```python
from build123d import *

# Parameters (mm, degrees)
SKETCH1_R                = 1.524
SKETCH1_R_2              = 1.27
SKETCH1_R_3              = 0.762
BOSS_EXTRUDE1_DEPTH      = 2.032
SKETCH1_3_R              = 1.27
SKETCH1_3_R_2            = 0.762
CUT_EXTRUDE1_DEPTH       = 1.524
SKETCH3_R                = 1.651
CUT_EXTRUDE2_DEPTH       = 0.254
SKETCH3_3_R              = 1.651
CUT_EXTRUDE3_DEPTH       = 2.032
SKETCH4_R                = 1.9685
BOSS_EXTRUDE2_DEPTH      = 0.254
BOSS_EXTRUDE3_DEPTH      = 2.54
BOSS_EXTRUDE3_DEPTH_BACK = 0.762
SKETCH4_3_R              = 1.9685
SKETCH4_3_R_2            = 1.651
SKETCH4_3_R_3            = 0.762
CUT_EXTRUDE4_DEPTH       = 2.032
SKETCH10_R               = 0.762
BOSS_EXTRUDE4_DEPTH      = 0.2286


with BuildPart() as part:
    # Sketch1 → Boss-Extrude1 (new body)
    # profile 1 of 7: a face of its own
    with BuildSketch(Plane(origin=(0, 0, 0), x_dir=(1, 0, 0), z_dir=(0, 1, 0))):
        with BuildLine():
            Line((2.032, -6.212875778), (2.032, -1.24150214))
            ThreePointArc((2.032, -1.24150214), (0, -2.38125), (-2.032, -1.24150214))
            Line((-2.032, -1.24150214), (-2.032, -6.206396707))
            ThreePointArc((-2.032, -6.206396707), (-0.877113637, -6.887720967), (0.461163405, -6.804175651))
            Line((0.461163405, -6.804175651), (2.032, -6.212875778))
        make_face()
        with Locations((0, -4.318)):
            Circle(SKETCH1_R, mode=Mode.SUBTRACT)
    # profile 2 of 7: a face of its own
    with BuildSketch(Plane(origin=(0, 0, 0), x_dir=(1, 0, 0), z_dir=(0, 1, 0))):
        with BuildLine():
            Line((2.032, 1.24150214), (2.032, 6.212875778))
            Line((2.032, 6.212875778), (0.461163405, 6.804175651))
            ThreePointArc((0.461163405, 6.804175651), (-0.877113637, 6.887720967), (-2.032, 6.206396707))
            Line((-2.032, 6.206396707), (-2.032, 1.24150214))
            ThreePointArc((-2.032, 1.24150214), (0, 2.38125), (2.032, 1.24150214))
        make_face()
        with Locations((0, 4.318)):
            Circle(SKETCH1_R, mode=Mode.SUBTRACT)
    # profile 3 of 7: a face of its own
    with BuildSketch(Plane(origin=(0, 0, 0), x_dir=(1, 0, 0), z_dir=(0, 1, 0))):
        with BuildLine():
            Line((2.032, -1.24150214), (2.032, 1.24150214))
            ThreePointArc((2.032, 1.24150214), (0, 2.38125), (-2.032, 1.24150214))
            Line((-2.032, 1.24150214), (-2.032, -1.24150214))
            ThreePointArc((-2.032, -1.24150214), (0, -2.38125), (2.032, -1.24150214))
        make_face()
    # profile 4 of 7: a face of its own
    with BuildSketch(Plane(origin=(0, 0, 0), x_dir=(1, 0, 0), z_dir=(0, 1, 0))):
        with Locations((0, -4.318)):
            Circle(SKETCH1_R)
        with Locations((0, -4.318)):
            Circle(SKETCH1_R_2, mode=Mode.SUBTRACT)
    # profile 5 of 7: a face of its own
    with BuildSketch(Plane(origin=(0, 0, 0), x_dir=(1, 0, 0), z_dir=(0, 1, 0))):
        with Locations((0, -4.318)):
            Circle(SKETCH1_R_2)
        with Locations(Location((0, -4.318, 0), (0, 0, 270))):
            Circle(SKETCH1_R_3, mode=Mode.SUBTRACT)
    # profile 6 of 7: a face of its own
    with BuildSketch(Plane(origin=(0, 0, 0), x_dir=(1, 0, 0), z_dir=(0, 1, 0))):
        with Locations((0, 4.318)):
            Circle(SKETCH1_R)
        with Locations((0, 4.318)):
            Circle(SKETCH1_R_2, mode=Mode.SUBTRACT)
    # profile 7 of 7: a face of its own
    with BuildSketch(Plane(origin=(0, 0, 0), x_dir=(1, 0, 0), z_dir=(0, 1, 0))):
        with Locations((0, 4.318)):
            Circle(SKETCH1_R_2)
        with Locations(Location((0, 4.318, 0), (0, 0, 270))):
            Circle(SKETCH1_R_3, mode=Mode.SUBTRACT)
    extrude(amount=BOSS_EXTRUDE1_DEPTH)

    # Sketch1<3> → Cut-Extrude1 (cut)
    # profile 1 of 2: a face of its own
    with BuildSketch(Plane(origin=(0, 0, 0), x_dir=(1, 0, 0), z_dir=(0, 1, 0))):
        with Locations(Location((0, -4.318, 0), (0, 0, 90))):
            Circle(SKETCH1_3_R)
        with Locations(Location((0, -4.318, 0), (0, 0, 270))):
            Circle(SKETCH1_3_R_2, mode=Mode.SUBTRACT)
    # profile 2 of 2: a face of its own
    with BuildSketch(Plane(origin=(0, 0, 0), x_dir=(1, 0, 0), z_dir=(0, 1, 0))):
        with Locations(Location((0, 4.318, 0), (0, 0, 90))):
            Circle(SKETCH1_3_R)
        with Locations(Location((0, 4.318, 0), (0, 0, 270))):
            Circle(SKETCH1_3_R_2, mode=Mode.SUBTRACT)
    extrude(amount=CUT_EXTRUDE1_DEPTH, mode=Mode.SUBTRACT)

    # Sketch3 → Cut-Extrude2 (cut)
    # profile 1 of 2: a face of its own
    with BuildSketch(Plane(origin=(0, 2.032, 0), x_dir=(1, 0, 0), z_dir=(0, 1, 0))):
        with BuildLine():
            Line((2.032, -1.24150214), (2.032, 1.24150214))
            ThreePointArc((2.032, 1.24150214), (0, 2.38125), (-2.032, 1.24150214))
            Line((-2.032, 1.24150214), (-2.032, -1.24150214))
            ThreePointArc((-2.032, -1.24150214), (0, -2.38125), (2.032, -1.24150214))
        make_face()
        Circle(SKETCH3_R, mode=Mode.SUBTRACT)
    # profile 2 of 2: a face of its own
    with BuildSketch(Plane(origin=(0, 2.032, 0), x_dir=(1, 0, 0), z_dir=(0, 1, 0))):
        Circle(SKETCH3_R)
    extrude(amount=-CUT_EXTRUDE2_DEPTH, mode=Mode.SUBTRACT)

    # Sketch3<3> → Cut-Extrude3 (cut)
    with BuildSketch(Plane(origin=(0, 2.032, 0), x_dir=(1, 0, 0), z_dir=(0, 1, 0))):
        with Locations(Location((0, 0, 0), (0, 0, 270))):
            Circle(SKETCH3_3_R)
    extrude(amount=-CUT_EXTRUDE3_DEPTH, mode=Mode.SUBTRACT)

    # Sketch4 → Boss-Extrude2 (add)
    with BuildSketch(Plane.XZ):
        with BuildLine():
            Line((2.032, -1.524), (2.032, 1.524))
            ThreePointArc((2.032, 1.524), (0, 2.54), (-2.032, 1.524))
            Line((-2.032, 1.524), (-2.032, -1.524))
            ThreePointArc((-2.032, -1.524), (0, -2.54), (2.032, -1.524))
        make_face()
        with Locations(Location((0, 0, 0), (0, 0, 270))):
            Circle(SKETCH4_R, mode=Mode.SUBTRACT)
    extrude(amount=BOSS_EXTRUDE2_DEPTH)

    # Sketch4<3> → Boss-Extrude3 (add, two sides: drawn at the far end of the back side and taken through both)
    # profile 1 of 2: a face of its own
    with BuildSketch(Plane.XZ.offset(-BOSS_EXTRUDE3_DEPTH_BACK)):
        with Locations(Location((0, 0, 0), (0, 0, 270))):
            Circle(SKETCH4_3_R)
        with Locations(Location((0, 0, 0), (0, 0, 90))):
            Circle(SKETCH4_3_R_2, mode=Mode.SUBTRACT)
    # profile 2 of 2: a face of its own
    with BuildSketch(Plane.XZ.offset(-BOSS_EXTRUDE3_DEPTH_BACK)):
        with Locations(Location((0, 0, 0), (0, 0, 90))):
            Circle(SKETCH4_3_R_2)
        with Locations(Location((0, 0, 0), (0, 0, 270))):
            Circle(SKETCH4_3_R_3, mode=Mode.SUBTRACT)
    extrude(amount=BOSS_EXTRUDE3_DEPTH + BOSS_EXTRUDE3_DEPTH_BACK)

    # Sketch6 → Cut-Extrude4 (cut)
    with BuildSketch(Plane.XZ):
        with BuildLine():
            Line((-2.032, 5.609449291), (-2.032, 6.206396707))
            ThreePointArc((-2.032, 6.206396707), (-0.003234375, 8.238399289), (2.032, 6.212875778))
            ThreePointArc((2.032, 6.212875778), (-0.031260659, 6.121699066), (-2.032, 5.609449291))
        make_face()
        with BuildLine():
            Line((-2.032, -5.784926759), (-2.032, -6.206396707))
            ThreePointArc((-2.032, -6.206396707), (-0.001969351, -7.444912354), (2.032, -6.212875778))
            ThreePointArc((2.032, -6.212875778), (-0.036162052, -6.342312682), (-2.032, -5.784926759))
        make_face()
    extrude(amount=-CUT_EXTRUDE4_DEPTH, mode=Mode.SUBTRACT)

    # Sketch10 → Boss-Extrude4 (add)
    # profile 1 of 2: a face of its own
    with BuildSketch(Plane(origin=(0, 2.032, 0), x_dir=(1, 0, 0), z_dir=(0, 1, 0))):
        with BuildLine():
            Line((-2.032, -1.24150214), (-2.032, -5.609449291))
            ThreePointArc((-2.032, -5.609449291), (-0.031260659, -6.121699066), (2.032, -6.212875778))
            Line((2.032, -6.212875778), (2.032, -1.24150214))
            ThreePointArc((2.032, -1.24150214), (0, -2.38125), (-2.032, -1.24150214))
        make_face()
        with Locations((0, -4.318)):
            Circle(SKETCH10_R, mode=Mode.SUBTRACT)
    # profile 2 of 2: a face of its own
    with BuildSketch(Plane(origin=(0, 2.032, 0), x_dir=(1, 0, 0), z_dir=(0, 1, 0))):
        with BuildLine():
            Line((-2.032, 5.784926759), (-2.032, 1.24150214))
            ThreePointArc((-2.032, 1.24150214), (0, 2.38125), (2.032, 1.24150214))
            Line((2.032, 1.24150214), (2.032, 6.212875778))
            ThreePointArc((2.032, 6.212875778), (-0.036162052, 6.342312682), (-2.032, 5.784926759))
        make_face()
        with Locations((0, 4.318)):
            Circle(SKETCH10_R, mode=Mode.SUBTRACT)
    extrude(amount=BOSS_EXTRUDE4_DEPTH)


solid = part.part
```
Geometry: final body of the model. Coordinates: model frame, mm. A direction names the side the tool comes from. Round coordinates to 2 decimals unless told otherwise and drop trailing zeros. Order: outer loops, then holes, each group sorted by start corner. A loop starts at its lowest first (then second) coordinate and runs counter-clockwise, first axis right, second up. Notation, with made-up numbers: (-39.75, -26.5) -> (10.25, -26.5) arc R32 cw to (10.25, 11.5) -> close; hole circle Ø2 at (-12, 46.5). An arc over 180 degrees is marked (long way). Use one line per item in the form item = value.
(1) Draft query along Z for faces 1 (the face through (-0.06, 0.75, -3.05)), 2 (the face through (-1, -0.254, 2)), 3 (the face through (-1.92, -1.38, 0.43)). Return one class per face: pulls with the +Z half, pulls with the -Z half, needs draft (parallel to the pull), parting line crosses it, or undercut.
Results list:
face_1 = undercut
face_2 = needs draft
face_3 = parting line crosses it
(2) Section A-A on z = 0. Return loops of the section in (x, y), and give its area (3 significant figures).
Results list:
outline = (-2.03, -0.25) -> (-1.97, -0.25) -> (-1.97, -2.54) -> (-0.76, -2.54) -> (-0.76, 0.76) -> (-1.65, 0.76) -> (-1.65, 1.78) -> (-2.03, 1.78) -> close; (0.76, -2.54) -> (1.97, -2.54) -> (1.97, -0.25) -> (2.03, -0.25) -> (2.03, 1.78) -> (1.65, 1.78) -> (1.65, 0.76) -> (0.76, 0.76) -> close
area = 8.87 mm^2
(3) Access query for faces 4 (the face through (0, 1.778, -2)), 5 (the face through (2.032, 1, 0)), 6 (the face through (-0.381, 0.751, 3.107)). Directions: +Z, -Z, +X, -X, +Y, -Y. A direction counts if a zero-diameter tool reaches every point of the face in a straight line with its end or side. Return the directions, or none.
Results list:
face_4 = +Y
face_5 = +Z, -Z, +X, +Y, -Y
face_6 = -Y
(4) Section D-D on z = 4. Return loops of the section in (x, y).
Results list:
outline = (-2.03, 0) -> (-1.23, 0) -> (-1.23, 1.52) -> (-0.69, 1.52) -> (-0.69, 2.26) -> (-2.03, 2.26) -> close; (0.69, 1.52) -> (1.23, 1.52) -> (1.23, 0) -> (2.03, 0) -> (2.03, 2.26) -> (0.69, 2.26) -> close
(5) Section C-C on y = -0.5. Return loops of the section in (x, z).
Results list:
outline = circle Ø3.94 at (0, 0); hole circle Ø1.52 at (0, 0)
(6) First-contact query: pin 1 Ø2 at (x, z) = (-1, 0) entering from +Y; pin 2 Ø0.9 at (x, z) = (0, 4.318) entering from -Y; pin 3 Ø2 at (x, z) = (0, -4.318) entering from +Y. Flat tips, straight axial feed; report the tip coordinate or a pass-through.
Results list:
pin_1 = 1.78
pin_2 = through
pin_3 = 2.26
(7) Ray query, probe 1 along X at (y, z) = (-1.4, 0); probe 2 along Z at (x, y) = (0, 1.7); probe 3 along Z at (x, y) = (0.45, 0.6). Return the intervals inside material, ascending. Write a range as [from, to].
Results list:
probe_1 = [-1.97, -0.76], [0.76, 1.97]
probe_2 = [-6.35, -5.08], [-3.56, -1.65], [1.65, 3.56], [5.08, 6.13]
probe_3 = [-6.37, -5.51], [-3.13, -0.61], [0.61, 3.13], [5.51, 6.18]
